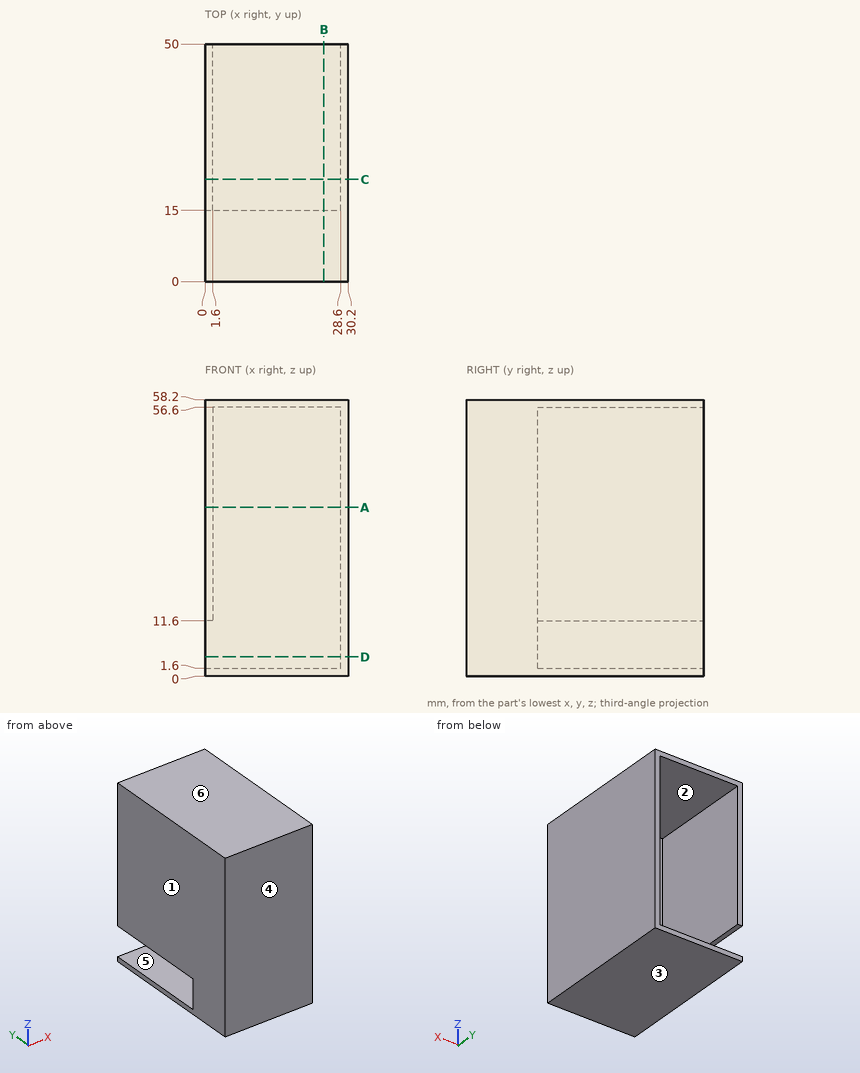
Geometry: see drawing. Coordinates: mm, zero at the bounding-box minimum. A direction names the side the tool comes from. Give positions to 0.01 mm unless a question says otherwise; leave off trailing zeros. Loops run counter-clockwise (first coordinate to the right, second up) from the corner with the lowest first, then second, coordinate; pieces in that order, holes last. Notation, with made-up numbers: (13.5, -30) -> (65.5, -30) arc R20 ccw to (65.5, 3) -> close; hole circle Ø2 at (18, 6). An arc over 180 degrees is marked (long way). Answer as a JSON object with one key per item and string values. Group by question number.
Item 1: Cut plane B-B, the plane x = 25. Return the cut outline in (y, z).
Item 2: Line query: probe 1 along X at (y, z) = (46.5, 29); probe 2 along Z at (x, y) = (16, 26); probe 3 along Y at (x, z) = (16.5, 30.5). Output: solid intervals per line, ascending.
Item 3: Cut plane C-C, the plane y = 21.5. Return the cut outline in (x, z).
Item 4: Pin query (flat end, axial travel): P1, Ø0.8, axis at x = 1, y = 26.5, coming from the -Z side; P2, Ø12, axis at x = 20, z = 12, coming from the +Y side. Return the tip coordinate at first contact, or that it passes through.
Item 5: Pull-direction query (Z, two-part tool) for the marked faces 3, 4, 5 and 6; classes: released by +Z, released by -Z, zero draft, split by the parting line, or undercut.
Item 6: Cut plane A-A, the plane z = 35.5. Return the cut outline in (x, y), and give its area (3 significant figures).
Item 7: Cut plane D-D, the plane z = 4. Return the cut outline in (x, y).
Item 8: Reachability of the marked faces 1 and 2 from +Z, -Z, +X, -X, +Y, -Y: full face, straight path, thin tool, end or side. Return the list, or none.
Checks:
{
 "1": {"outline": "(0, 0) -> (50, 0) -> (50, 1.6) -> (15, 1.6) -> (15, 56.6) -> (50, 56.6) -> (50, 58.2) -> (0, 58.2) -> close"},
 "2": {"probe 1": "x = 0 to 1.6, 28.6 to 30.2", "probe 2": "z = 0 to 1.6, 56.6 to 58.2", "probe 3": "y = 0 to 15"},
 "3": {"outline": "(0, 0) -> (30.2, 0) -> (30.2, 58.2) -> (0, 58.2) -> (0, 11.6) -> (1.6, 11.6) -> (1.6, 56.6) -> (28.6, 56.6) -> (28.6, 1.6) -> (0, 1.6) -> close"},
 "4": {"P1": "stops at z = 0", "P2": "stops at y = 15"},
 "5": {"face 3": "released by -Z", "face 4": "zero draft", "face 5": "undercut", "face 6": "released by +Z"},
 "6": {"outline": "(0, 0) -> (30.2, 0) -> (30.2, 50) -> (28.6, 50) -> (28.6, 15) -> (1.6, 15) -> (1.6, 50) -> (0, 50) -> close", "area": "565 mm²"},
 "7": {"outline": "(0, 0) -> (30.2, 0) -> (30.2, 50) -> (28.6, 50) -> (28.6, 15) -> (0, 15) -> close"},
 "8": {"face 1": "+Z, -Z, -X, +Y, -Y", "face 2": "+Y"}
}
